Source: CAD feature listing. Evaluate the final solid. Frame: model axes, mm. A direction names the side the tool comes from. Round coordinates to 2 decimals unless told otherwise and drop trailing zeros. Loops run counter-clockwise (first coordinate to the right, second up) from the corner with the lowest first, then second, coordinate; pieces in that order, holes last. Notation, with made-up numbers: (-4, 70.25) -> (3, 70.25) arc R19 cw to (3, 106.25) -> close; hole circle Ø11 at (9.5, 19.25). An arc over 180 degrees is marked (long way). Put each result on its own line as item: value. Start each with the question number.
1. Material intervals for L1, parallel to Y at x = 12, z = 21; L2, parallel to Z at x = 20, y = -17.9; L3, parallel to Y at x = 30, z = 3.65, sorted ascending.
2. Cut plane B-B (z = 27.5). Return the cut outline in (x, y), then the cut area to 3 significant figures.
3. Draft query along Y for faces 3 (the flat face through (20, -5, 18)), 4 (the flat face through (20, 0, 15)), 5 (the cylindrical face through (31.27, -10.97, 2.46)), 6 (the flat face through (0, -10, 2)). Return one class per face: pulls with the +Y half, pulls with the -Y half, needs draft (parallel to the pull), parting line crosses it, or undercut.
4. Set-up query: faces 1 (the flat face through (20, -20, 15)), 2 (the flat face through (20, -15, 18)). Return all of +Z, -Z, +X, -X, +Y, -Y with unobstructed straight access to the full face (end or side cutting, diameter ignored); none if empty.
5. Cut plane A-A (y = -4). Return the cut outline in (x, z).
6. Contact query for flat-ended pins moving along their axis: pin 1 (5 mm diameter, centred on y = -7, z = 17.5, fed in from +X); pin 2 (3 mm diameter, centred on x = 19, z = 22, fed in from +Y); pin 3 (3 mm diameter, centred on x = 22.5, y = -8, fed in from +Z); pin 4 (6 mm diameter, centred on y = -18, z = 8.5, fed in from -X). Output: stop coordinate, or through.
7. Cut plane C-C (x = 20). Return the cut outline in (y, z).
8. Cut plane D-D (z = 35). Return the cut outline in (x, y).
```python
from build123d import *

# Parameters (mm, degrees)
F3_R     = 2.55
F4_DEPTH = 5
F0_W     = 40
F0_H     = 5
F5_DEPTH = 5
F6_D     = 3.2


with BuildPart() as f4:
    # F3 (on Front) → F4 (new body)
    with BuildSketch(Plane.XZ):
        with BuildLine():
            Line((0, 5), (0, 0))
            Line((0, 0), (40, 0))
            Line((40, 0), (40, 5))
            Line((40, 5), (31.9607029074, 30.3005375883))
            ThreePointArc((31.9607029074, 30.3005375883), (20, 39.05), (8.0392970926, 30.3005375883))
            Line((8.0392970926, 30.3005375883), (0, 5))
        make_face()
        with Locations((20, 26.5)):
            Circle(F3_R, mode=Mode.SUBTRACT)
    extrude(amount=F4_DEPTH)

    # F0 (on face) → F5 (join)
    with BuildSketch(Plane.XZ.offset(5)):
        with Locations((20, 2.5)):
            Rectangle(F0_W, F0_H)
    extrude(amount=F5_DEPTH)

    # F1: F4 across face


with BuildPart() as f4_1:
    add(f4.part)
    add(f4.part.mirror(Plane(origin=(20, -10, 2.5), x_dir=(1, 0, 0), z_dir=(0, -1, 0))))

    # F6 (through all)
    with Locations(Plane.XY.offset(5)):
        with Locations((10, -10), (30, -10)):
            Hole(F6_D / 2)


solid = f4_1.part
```
Solution:
1. L1: y = -20 to -15, -5 to 0
1. L2: z = 0 to 23.95, 29.05 to 39.05
1. L3: y = -20 to -11.6, -8.4 to 0
2. outline: (7.15, -20) -> (17.65, -20) -> (17.65, -15) -> (7.15, -15) -> close; (7.15, -5) -> (17.65, -5) -> (17.65, 0) -> (7.15, 0) -> close; (22.35, -20) -> (32.85, -20) -> (32.85, -15) -> (22.35, -15) -> close; (22.35, -5) -> (32.85, -5) -> (32.85, 0) -> (22.35, 0) -> close
2. area: 210 mm^2
3. face 3: undercut
3. face 4: pulls with the +Y half
3. face 5: undercut
3. face 6: needs draft
4. face 1: +Z, -Z, +X, -X, -Y
4. face 2: +Z, +X, -X
5. outline: (0, 0) -> (40, 0) -> (40, 5) -> (31.96, 30.3) arc R12.55 ccw to (8.04, 30.3) -> (0, 5) -> close; hole circle Ø5.1 at (20, 26.5)
6. pin 1: stops at x = 36.5
6. pin 2: stops at y = 0
6. pin 3: stops at z = 5
6. pin 4: stops at x = 0.16
7. outline: (-20, 0) -> (0, 0) -> (0, 23.95) -> (-5, 23.95) -> (-5, 5) -> (-15, 5) -> (-15, 23.95) -> (-20, 23.95) -> close; (-20, 29.05) -> (-15, 29.05) -> (-15, 39.05) -> (-20, 39.05) -> close; (-5, 29.05) -> (0, 29.05) -> (0, 39.05) -> (-5, 39.05) -> close
8. outline: (10.77, -20) -> (29.23, -20) -> (29.23, -15) -> (10.77, -15) -> close; (10.77, -5) -> (29.23, -5) -> (29.23, 0) -> (10.77, 0) -> close
